Job drawing, mm, ordinate dimensions from the low corner. One solid piece. A direction names the side the tool comes from. Give positions to 0.01 mm unless a question says otherwise; leave off trailing zeros. Loops run counter-clockwise (first coordinate to the right, second up) from the corner with the lowest first, then second, coordinate; pieces in that order, holes last. Notation, with made-up numbers: (47.25, 52.5) -> (59.25, 52.5) arc R26 ccw to (59.25, 66.5) -> close; hole circle Ø4 at (-1, -12.5). An arc over 180 degrees is marked (long way). Answer as a JSON object with one key per item and string values. Group by question number.
Q1. Band-saw the part on D-D, the plane y = 19. Write the cut outline in (x, z), plus the area to 3 significant figures.
Q2. Drop flat-ended pins along their axis: pin 1 (4 mm diameter, centred on y = 68, z = 8.85, fed in from +X); pin 2 (6 mm diameter, centred on y = 22, z = 11.5, fed in from +X); pin 3 (5.5 mm diameter, centred on x = 55.5, z = 5, fed in from +Y); pin 4 (4 mm diameter, centred on y = 67, z = 4.5, fed in from +X). Give the stop position or say it passes through.
Q3. Band-saw the part on B-B, the plane y = 39.65. Write the cut outline in (x, z).
Q4. Wall check: probe 1 along Y at (x, z) = (2.5, 8.85); probe 2 along Z at (x, y) = (6.5, 68); probe 3 along Y at (x, z) = (33, 9). Give the ranges that are in metal, low to high. Write a range as from..to.
Q5. Band-saw the part on C-C, the plane z = 8.85. Write the cut outline in (x, y).
Q6. Tool access for the marked faces 1 and 2: list every direction of +Z, -Z, +X, -X, +Y, -Y with a clear straight run to the whole face (end or side of a thin tool).
Q7. Band-saw the part on A-A, the plane x = 67. Write the cut outline in (y, z).
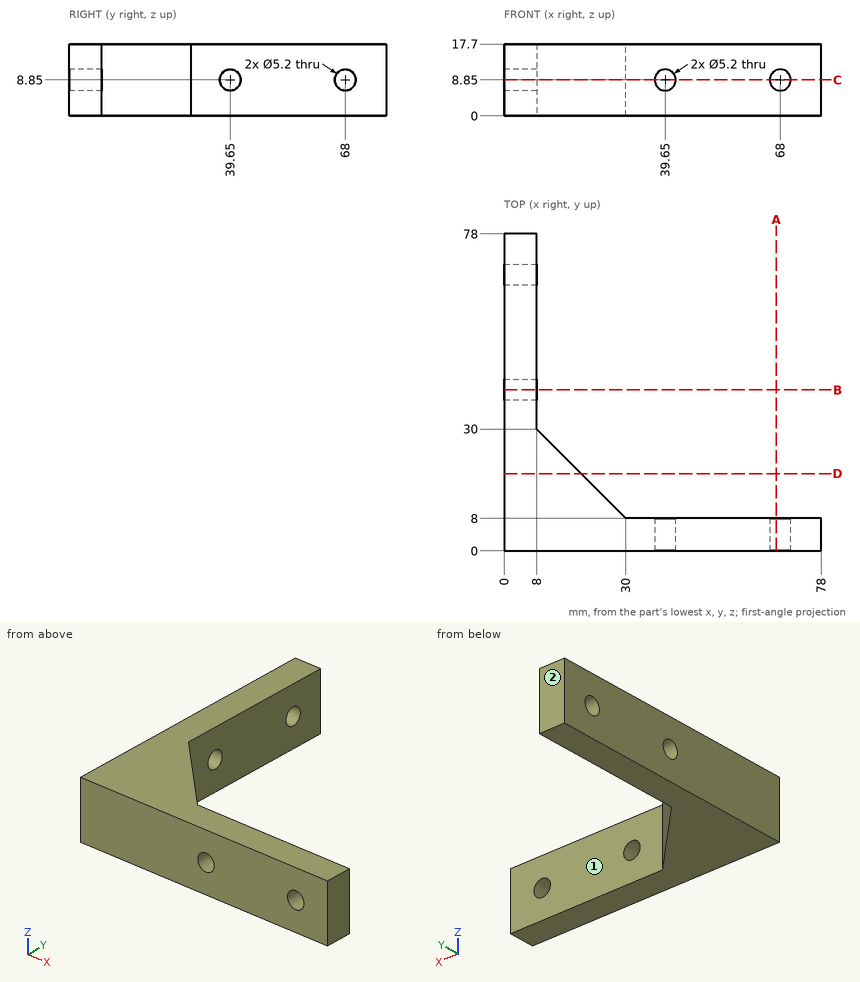
Worked answers:
{
 "1": {"outline": "(0, 0) -> (19, 0) -> (19, 17.7) -> (0, 17.7) -> close", "area": "336 mm2"},
 "2": {"pin 1": "through", "pin 2": "x = 19", "pin 3": "y = 8", "pin 4": "x = 8"},
 "3": {"outline": "(0, 0) -> (8, 0) -> (8, 6.25) -> (0, 6.25) -> close; (0, 11.45) -> (8, 11.45) -> (8, 17.7) -> (0, 17.7) -> close"},
 "4": {"probe 1": "0..37.05, 42.25..65.4, 70.6..78", "probe 2": "0..6.25, 11.45..17.7", "probe 3": "0..8"},
 "5": {"outline": "(0, 0) -> (37.05, 0) -> (37.05, 8) -> (30, 8) -> (8, 30) -> (8, 37.05) -> (0, 37.05) -> close; (0, 42.25) -> (8, 42.25) -> (8, 65.4) -> (0, 65.4) -> close; (0, 70.6) -> (8, 70.6) -> (8, 78) -> (0, 78) -> close; (42.25, 0) -> (65.4, 0) -> (65.4, 8) -> (42.25, 8) -> close; (70.6, 0) -> (78, 0) -> (78, 8) -> (70.6, 8) -> close"},
 "6": {"face 1": "+Z, -Z, +X, +Y", "face 2": "+Z, -Z, +X, -X, +Y"},
 "7": {"outline": "(0, 0) -> (8, 0) -> (8, 6.45) -> (0, 6.45) -> close; (0, 11.25) -> (8, 11.25) -> (8, 17.7) -> (0, 17.7) -> close"}
}
